```python
from build123d import *

# Parameters (mm, degrees)
F1_DEPTH = 300
F2_R     = 90
F2_W     = 367.9086971283
F2_H     = 300
F3_DEPTH = 501
F4_W     = 155
F4_H     = 160
F5_DEPTH = 501
F6_R     = 100
F7_DEPTH = 100


with BuildPart() as f1:
    # F0 (on Top) → F1 (new body)
    with BuildSketch(Plane.XY):
        with BuildLine():
            Line((-82.5, -150), (82.5, -150))
            ThreePointArc((82.5, -150), (232.5, 0), (82.5, 150))
            Line((82.5, 150), (-82.5, 150))
            ThreePointArc((-82.5, 150), (-232.5, 0), (-82.5, -150))
        make_face()
    extrude(amount=F1_DEPTH)

    # F2 (on face) → F3 (cut)
    with BuildSketch(Plane(origin=(0, 0, 0), x_dir=(1, 0, 0), z_dir=(0, 0, -1))):
        with Locations((82.5, 0)):
            Circle(F2_R)
        with Locations((-266.4543485641, 0)):
            Rectangle(F2_W, F2_H)
    extrude(amount=-F3_DEPTH, mode=Mode.SUBTRACT)

    # F4 (on face) → F5 (cut)
    with BuildSketch(Plane.XZ.offset(150)):
        with Locations((160, 150)):
            Rectangle(F4_W, F4_H)
        with Locations((5, 150)):
            Rectangle(F4_W, F4_H)
    extrude(amount=-F5_DEPTH, mode=Mode.SUBTRACT)

    # F6 (on face) → F7 (join)
    with BuildSketch(Plane(origin=(-82.5, 0, 0), x_dir=(0, -1, 0), z_dir=(-1, 0, 0))):
        with Locations((35, 150)):
            Circle(F6_R)
    extrude(amount=F7_DEPTH)


solid = f1.part
```
Design review of the part built by this model. Coordinates are the model's own, in mm. A direction names the side the tool comes from. Round coordinates to 2 decimals unless told otherwise and drop trailing zeros. Order: outer loops, then holes, each group sorted by start corner. A loop starts at its lowest first (then second) coordinate and runs counter-clockwise, first axis right, second up. Notation, with made-up numbers: (-37.5, 45.25) - (-28.5, 45.25) arc R12 ccw to (-28.5, 67.25) - close; hole circle Ø8 at (21.25, 3.25). An arc over 180 degrees is marked (long way). Return JSON: item names as keys, results as strings.
Q1. Machinability: for faces 1 (the flat face through (-72.5, -2, 149)), 2 (the flat face through (-74, -150, 148)), 3 (the flat face through (-82.5, 69, 148)), which of the approach directions +Z, -Z, +X, -X, +Y, -Y give a long, thin tool a straight path to every point of the face, cutting with its end or side? Answer none if there is none.
Computed values:
{"face 1": "+X, +Y, -Y", "face 2": "+Z, -Z, +X, -X, -Y", "face 3": "-X"}
Q2. Consider section C-C on z = 235. Write out the cut boundary in (x, y), plus the area to 3 significant figures.
Computed values:
{"outline": "(-182.5, -87.68) - (-82.5, -87.68) - (-82.5, -150) - (82.5, -150) arc R150 ccw to (82.5, 150) - (-82.5, 150) - (-82.5, 17.68) - (-182.5, 17.68) - close; hole circle Ø180 at (82.5, 0)", "area": "69,900 mm2"}
Q3. Consider section D-D on x = 30. Write out the cut boundary in (y, z), plus the area to 3 significant figures.
Computed values:
{"outline": "(-150, 0) - (-73.1, 0) - (-73.1, 70) - (-150, 70) - close; (-150, 230) - (-73.1, 230) - (-73.1, 300) - (-150, 300) - close; (73.1, 0) - (150, 0) - (150, 70) - (73.1, 70) - close; (73.1, 230) - (150, 230) - (150, 300) - (73.1, 300) - close", "area": "21,500 mm2"}
Q4. Consider section A-A on x = -35. Write out the cut boundary in (y, z), plus the area to 3 significant figures.
Computed values:
{"outline": "(-150, 0) - (150, 0) - (150, 70) - (-150, 70) - close; (-150, 230) - (150, 230) - (150, 300) - (-150, 300) - close", "area": "42,000 mm2"}
Q5. The part is to be moulded in two halves that separate along Y. For faces 4 (the cylindrical face through (11.079, 54.764, 264.51)), 5 (the flat face through (3, 69, 300)), 6 (the cylindrical face through (11.079, 54.764, 34.51)), 7 (the flat face through (1, 150, 48)), say which applies: pulls with the +Y half, pulls with the -Y half, needs draft (parallel to the pull), parting line crosses it, or undercut.
Computed values:
{"face 4": "undercut", "face 5": "needs draft", "face 6": "undercut", "face 7": "pulls with the +Y half"}
Q6. Consider section B-B on y = -35. Write out the cut boundary in (x, z).
Computed values:
{"outline": "(-182.5, 50) - (-82.5, 50) - (-82.5, 0) - (-0.42, 0) - (-0.42, 70) - (-72.5, 70) - (-72.5, 230) - (-0.42, 230) - (-0.42, 300) - (-82.5, 300) - (-82.5, 250) - (-182.5, 250) - close; (165.42, 0) - (228.36, 0) - (228.36, 70) - (165.42, 70) - close; (165.42, 230) - (228.36, 230) - (228.36, 300) - (165.42, 300) - close"}
Q7. Wall thickness on L1, parallel to Z at x = 59, y = 102.5; L2, parallel to Y at x = 82.5, z = 283; L3, parallel to X at y = 0, z = 284: over which ranges is each line inside the solid? List them lowest first. Write a range as [from, to].
Computed values:
{"L1": "z = [0, 70], [230, 300]", "L2": "y = [-150, -90], [90, 150]", "L3": "x = [-82.5, -7.5], [172.5, 232.5]"}
Q8. For pin 1 Ø5 at (x, y) = (-111, 7) entering from -Z; pin 2 Ø3 at (y, z) = (78, 227.5) entering from +X; pin 3 Ø1.5 at (x, y) = (159.5, -70.5) entering from -Z; pin 4 Ø1.5 at (x, y) = (-124, -113) entering from +Z, all flat-tipped, find the tip position at first contact; note any pin that passes through.
Computed values:
{"pin 1": "stops at z = 58.13", "pin 2": "stops at x = -72.5", "pin 3": "stops at z = 0", "pin 4": "stops at z = 213.5"}
